The model under review builds one solid part; all positions refer to its coordinate system, in mm. A direction names the side the tool comes from. Round coordinates to 2 decimals unless told otherwise and drop trailing zeros. Write each loop counter-clockwise with the first axis right and the second up, starting at its lowest first coordinate (ties: lowest second). Pieces come first, ordered by that corner, then holes.
Item 1: Clearance check with flat-ended pins moving along their axes: pin 1 Ø5.5 at (x, y) = (28, -1.5) entering from +Z; pin 2 Ø1.5 at (x, y) = (27.5, 0.5) entering from -Z; pin 3 Ø2.5 at (x, y) = (-28, -0.5) entering from +Z; pin 4 Ø1.5 at (x, z) = (15, 4) entering from -Y. State where each tip first meets the part, or that it passes through.
Item 2: Draft analysis for pull direction Y (two halves, no side actions). For faces 3 (the face through (26.719, 4.783, 7.133)), 4 (the face through (30.083, -3.188, 10.884)), 5 (the face through (-34.93, 6.9, 1.01)), 6 (the face through (-28, 0, 2)), state which applies: +Y half, -Y half, draft (parallel to the pull), parting line (faces both ways), or undercut.
Item 3: Add section B-B (z = 9). State how many separate pieces and enclosed holes the cut face has, plus the area to 3 significant figures.
Item 4: Machinability: for faces 1 (the face through (-35.5, 0, 1)), 2 (the face through (27, 0, 2)), which of the approach directions +Z, -Z, +X, -X, +Y, -Y give a long, thin tool a straight path to every point of the face, cutting with its end or side? Answer none if there is none.
Item 5: To check wall thickness, follow L1, parallel to X at y = 0.25, z = 11.25; L2, parallel to X at y = 0, z = 7; L3, parallel to Y at x = -26, z = 1. State the ranges of each line that lie inside material, in increasing order.
Item 6: Add section A-A (x = -10). Give the boundary of the cut face in (y, z), plus the area to 3 significant figures.
```python
from build123d import *

# Parameters (mm, degrees)
F0_W          = 71
F0_H          = 15
F1_DEPTH      = 2
F2_R          = 2
F4_R          = 6
F4_R_2        = 2.55
F5_DEPTH      = 8
F5_DEPTH_BACK = 2.3


with BuildPart() as f1:
    # F0 (on Top) → F1 (new body)
    with BuildSketch(Plane.XY):
        Rectangle(F0_W, F0_H)
    extrude(amount=F1_DEPTH)

    # F2
    f2_edges = [f1.edges().sort_by_distance(p)[0] for p in [
        (-35.5, 7.5, 1),
        (-35.5, -7.5, 1),
        (35.5, -7.5, 1),
        (35.5, 7.5, 1),
    ]]
    fillet(f2_edges, radius=F2_R)

    # F4 (on face) → F5 (join, two sides)
    with BuildSketch(Plane(origin=(0, -0.568173, 3.222268), x_dir=(1, 0, 0), z_dir=(0, -0.173648, 0.984808))) as f5_sk:
        with Locations((-27.5, 0)):
            Circle(F4_R)
        with Locations((-27.5, 0)):
            Circle(F4_R_2, mode=Mode.SUBTRACT)
        with Locations((27.5, 0)):
            Circle(F4_R)
        with Locations((27.5, 0)):
            Circle(F4_R_2, mode=Mode.SUBTRACT)
    extrude(amount=F5_DEPTH)
    extrude(f5_sk.sketch, amount=-F5_DEPTH_BACK)


solid = f1.part
```
Numbers:
1. pin 1: stops at z = 11.67
1. pin 2: stops at z = 0
1. pin 3: stops at z = 11.58
1. pin 4: passes through
2. face 3: parting line
2. face 4: -Y half
2. face 5: +Y half
2. face 6: undercut
3. separate pieces: 2
3. enclosed holes: 2
3. area: 188 mm2
4. face 1: +Z, -Z, -X, +Y, -Y
4. face 2: none
5. L1: x = -33.08 to -28.79, -26.21 to -21.92, 21.92 to 26.21, 28.79 to 33.08
5. L2: x = -33.38 to -29.74, -25.26 to -21.62, 21.62 to 25.26, 29.74 to 33.38
5. L3: y = -7.5 to 7.5
6. outline: (-7.5, 0) - (7.5, 0) - (7.5, 2) - (-7.5, 2) - close
6. area: 30.0 mm2
